Verification items for the finished model (mm, model axes). A direction names the side the tool comes from. Round coordinates to 2 decimals unless told otherwise and drop trailing zeros. Order: outer loops, then holes, each group sorted by start corner. A loop starts at its lowest first (then second) coordinate and runs counter-clockwise, first axis right, second up. Notation, with made-up numbers: (6.5, 0.5) -> (54.5, 0.5) arc R19 cw to (54.5, 10.5) -> close; hole circle Ø6 at (88.25, 81.5). An arc over 180 degrees is marked (long way). Put each result on its own line as item: value.
from build123d import *

# Parameters (mm, degrees)
F0_W     = 812.8
F0_H     = 812.8
F0_R     = 55
F0_R_2   = 82.5
F1_DEPTH = 100
F2_W     = 67.6
F2_H     = 150
F3_DEPTH = 120
F4_R     = 50
F5_R     = 37.5
F6_DEPTH = 547.801


with BuildPart() as f1:
    # F0 (on Front) → F1 (new body)
    with BuildSketch(Plane.XZ):
        Rectangle(F0_W, F0_H)
        with Locations((-271.4, -271.4)):
            Circle(F0_R, mode=Mode.SUBTRACT)
        Circle(F0_R_2, mode=Mode.SUBTRACT)
        with Locations((271.4, -271.4)):
            Circle(F0_R, mode=Mode.SUBTRACT)
        with Locations((-271.4, 271.4)):
            Circle(F0_R, mode=Mode.SUBTRACT)
        with Locations((271.4, 271.4)):
            Circle(F0_R, mode=Mode.SUBTRACT)
    extrude(amount=F1_DEPTH)

    # F2 (on face) → F3 (join)
    with BuildSketch(Plane.XZ.offset(100)):
        with Locations((-107.6, 326.4)):
            Rectangle(F2_W, F2_H)
        with Locations((0, 326.4)):
            Rectangle(F2_W, F2_H)
        with Locations((107.6, 326.4)):
            Rectangle(F2_W, F2_H)
        with Locations((107.6, -326.4)):
            Rectangle(F2_W, F2_H)
        with Locations((-107.6, -326.4)):
            Rectangle(F2_W, F2_H)
        with Locations((0, -326.4)):
            Rectangle(F2_W, F2_H)
    extrude(amount=F3_DEPTH)

    # F4
    f4_edges = [f1.edges().sort_by_distance(p)[0] for p in [
        (107.6, -220, -401.4),
        (0, -220, -401.4),
        (-107.6, -220, -401.4),
        (-107.6, -220, -251.4),
        (0, -220, -251.4),
        (107.6, -220, -251.4),
        (107.6, -220, 251.4),
        (107.6, -220, 401.4),
        (0, -220, 251.4),
        (0, -220, 401.4),
        (-107.6, -220, 401.4),
        (-107.6, -220, 251.4),
    ]]
    fillet(f4_edges, radius=F4_R)

    # F5 (on face) → F6 (cut, through all)
    with BuildSketch(Plane.YZ.offset(141.4)):
        with Locations((-175, -326.4)):
            Circle(F5_R)
        with Locations((-175, 326.4)):
            Circle(F5_R)
    extrude(amount=-F6_DEPTH, mode=Mode.SUBTRACT)


solid = f1.part
Item 1: Section check B-B on y = -120. Record the boundary of the cut face in (x, z).
Check sheet entries:
outline: (-141.4, -401.4) -> (-73.8, -401.4) -> (-73.8, -251.4) -> (-141.4, -251.4) -> close; (-141.4, 251.4) -> (-73.8, 251.4) -> (-73.8, 401.4) -> (-141.4, 401.4) -> close; (-33.8, -401.4) -> (33.8, -401.4) -> (33.8, -251.4) -> (-33.8, -251.4) -> close; (-33.8, 251.4) -> (33.8, 251.4) -> (33.8, 401.4) -> (-33.8, 401.4) -> close; (73.8, -401.4) -> (141.4, -401.4) -> (141.4, -251.4) -> (73.8, -251.4) -> close; (73.8, 251.4) -> (141.4, 251.4) -> (141.4, 401.4) -> (73.8, 401.4) -> close
Item 2: Release check for a two-part mould opening along X. For faces 6 (the flat face through (-33.8, -132, 325)), 7 (the cylindrical face through (108.073, -204.964, -387.142)), 8 (the flat face through (-406.4, -49, -6)) record: +X half, -X half, draft (parallel to the pull), parting line (faces both ways), or undercut.
Check sheet entries:
face 6: undercut
face 7: draft
face 8: -X half
Item 3: Tool access check on faces 1 (the flat face through (-73.8, -132, -327)), 2 (the flat face through (-141.4, -132, 325)), 3 (the flat face through (-108, -220, 327)), 4 (the flat face through (107, -135, -401.4)), 5 (the cylindrical face through (108.073, -204.964, -265.658)). Record the directions out of +Z, -Z, +X, -X, +Y, -Y that give a thin tool (end or side, any length) a straight path to the whole face; none if there is none.
Check sheet entries:
face 1: +Z, -Z, -Y
face 2: +Z, -Z, -X, -Y
face 3: +Z, -Z, +X, -X, -Y
face 4: -Z, +X, -X, -Y
face 5: +X, -X, -Y
Item 4: Section check C-C on y = -37. Record the boundary of the cut face in (x, z).
Check sheet entries:
outline: (-406.4, -406.4) -> (406.4, -406.4) -> (406.4, 406.4) -> (-406.4, 406.4) -> close; hole circle Ø110 at (-271.4, -271.4); hole circle Ø110 at (-271.4, 271.4); hole circle Ø165 at (0, 0); hole circle Ø110 at (271.4, -271.4); hole circle Ø110 at (271.4, 271.4)
Item 5: Material ranges on L1, parallel to Z at x = -271.4, y = -47; L2, parallel to X at y = -109, z = -322; L3, parallel to X at y = -70.5, z = 241.5, recorded low to high. Write a range as [from, to].
Check sheet entries:
L1: z = [-406.4, -326.4], [-216.4, 216.4], [326.4, 406.4]
L2: x = [-141.4, -73.8], [-33.8, 33.8], [73.8, 141.4]
L3: x = [-406.4, -317.56], [-225.24, 225.24], [317.56, 406.4]
Item 6: Section check A-A on x = 0. Record the boundary of the cut face in (y, z), then the cut area to 3 significant figures.
Check sheet entries:
outline: (-220, -351.4) arc R50 ccw to (-170, -401.4) -> (-100, -401.4) -> (-100, -406.4) -> (0, -406.4) -> (0, -82.5) -> (-100, -82.5) -> (-100, -251.4) -> (-170, -251.4) arc R50 ccw to (-220, -301.4) -> close; (-220, 301.4) arc R50 ccw to (-170, 251.4) -> (-100, 251.4) -> (-100, 82.5) -> (0, 82.5) -> (0, 406.4) -> (-100, 406.4) -> (-100, 401.4) -> (-170, 401.4) arc R50 ccw to (-220, 351.4) -> close; hole circle Ø75 at (-175, -326.4); hole circle Ø75 at (-175, 326.4)
area: 89,800 mm^2
Item 7: Gauge pin test, flat end, axial feed: pin 1 Ø20.5 at (x, y) = (-113, -151.5) entering from +Z. Record the tip position at first contact, or that the pin passes through.
Check sheet entries:
pin 1: stops at z = 401.4
Item 8: Section check D-D on x = -271.4. Record the boundary of the cut face in (y, z), then the cut area to 3 significant figures.
Check sheet entries:
outline: (-100, -406.4) -> (0, -406.4) -> (0, -326.4) -> (-100, -326.4) -> close; (-100, -216.4) -> (0, -216.4) -> (0, 216.4) -> (-100, 216.4) -> close; (-100, 326.4) -> (0, 326.4) -> (0, 406.4) -> (-100, 406.4) -> close
area: 59,300 mm^2
